from build123d import *

# Parameters (mm, degrees)
F0_R     = 11
F1_DEPTH = 1


with BuildPart() as f1:
    # F0 (on Top) → F1 (new body)
    with BuildSketch(Plane.XY):
        with BuildLine():
            ThreePointArc((8.291562, -12.5), (15, 0), (8.291562, 12.5))
            ThreePointArc((8.291562, 12.5), (0, 40), (-8.291562, 12.5))
            ThreePointArc((-8.291562, 12.5), (-15, 0), (-8.291562, -12.5))
            ThreePointArc((-8.291562, -12.5), (0, -40), (8.291562, -12.5))
        make_face()
        with BuildLine():
            ThreePointArc((0, -14), (7.778175, -17.221825), (11, -25))
            ThreePointArc((11, -25), (-7.778175, -32.778175), (0, -14))
        make_face(mode=Mode.SUBTRACT)
        Circle(F0_R, mode=Mode.SUBTRACT)
        with Locations((0, 25)):
            Circle(F0_R, mode=Mode.SUBTRACT)
    extrude(amount=F1_DEPTH)


solid = f1.part
Design review of the part built by this model. Coordinates are the model's own, in mm. Round coordinates to 2 decimals unless told otherwise and drop trailing zeros. Write each loop counter-clockwise with the first axis right and the second up, starting at its lowest first coordinate (ties: lowest second). Pieces come first, ordered by that corner, then holes.
Item 1: Consider section D-D on x = 1. Give the boundary of the cut face in (y, z).
Item 2: Consider section C-C on z = 0.85. Give the boundary of the cut face in (x, y).
Item 3: Consider section A-A on x = 12. Give the boundary of the cut face in (y, z), and give its area (3 significant figures).
Item 4: Wall thickness on L1, parallel to Y at x = 0, z = 0.8; L2, parallel to Y at x = -2.5, z = 0.95; L3, parallel to X at y = -25, z = 0.45: over which ranges is each line inside the solid? List them lowest first.
Item 5: For pin 1 Ø2 at (x, y) = (3, -8.5) entering from +Z, flat-tipped, find the tip position at first contact; note if it passes through.
Item 6: Draft analysis for pull direction X (two halves, no side actions). For faces 1 (the flat face through (-7, -9, 1)), 2 (the cylindrical face through (-2.38, 14.26, 0.49)), state which applies: released by +X, released by -X, zero draft, split by the parting line, or undercut.
Item 7: Consider section B-B on y = 0. Give the boundary of the cut face in (x, z), and give its area (3 significant figures).
Check values:
1. outline: (-39.97, 0) - (-35.95, 0) - (-35.95, 1) - (-39.97, 1) - close; (-14.05, 0) - (-10.95, 0) - (-10.95, 1) - (-14.05, 1) - close; (10.95, 0) - (14.05, 0) - (14.05, 1) - (10.95, 1) - close; (35.95, 0) - (39.97, 0) - (39.97, 1) - (35.95, 1) - close
2. outline: (-8.29, -12.5) arc R15 ccw (long way) to (8.29, -12.5) arc R15 ccw to (8.29, 12.5) arc R15 ccw (long way) to (-8.29, 12.5) arc R15 ccw to start; hole circle Ø22 at (0, 0); hole circle Ø22 at (0, 25); hole (0, -14) arc R11 ccw (long way) to (11, -25) arc R11 ccw to start
3. outline: (-34, 0) - (-16, 0) - (-16, 1) - (-34, 1) - close; (-9, 0) - (9, 0) - (9, 1) - (-9, 1) - close; (16, 0) - (34, 0) - (34, 1) - (16, 1) - close
3. area: 54.0 mm2
4. L1: y = -40 to -36, -14 to -11, 11 to 14, 36 to 40
4. L2: y = -39.79 to -35.71, -14.29 to -10.71, 10.71 to 14.29, 35.71 to 39.79
4. L3: x = -15 to -11, 11 to 15
5. pin 1: passes through
6. face 1: zero draft
6. face 2: undercut
7. outline: (-15, 0) - (-11, 0) - (-11, 1) - (-15, 1) - close; (11, 0) - (15, 0) - (15, 1) - (11, 1) - close
7. area: 8.00 mm2
